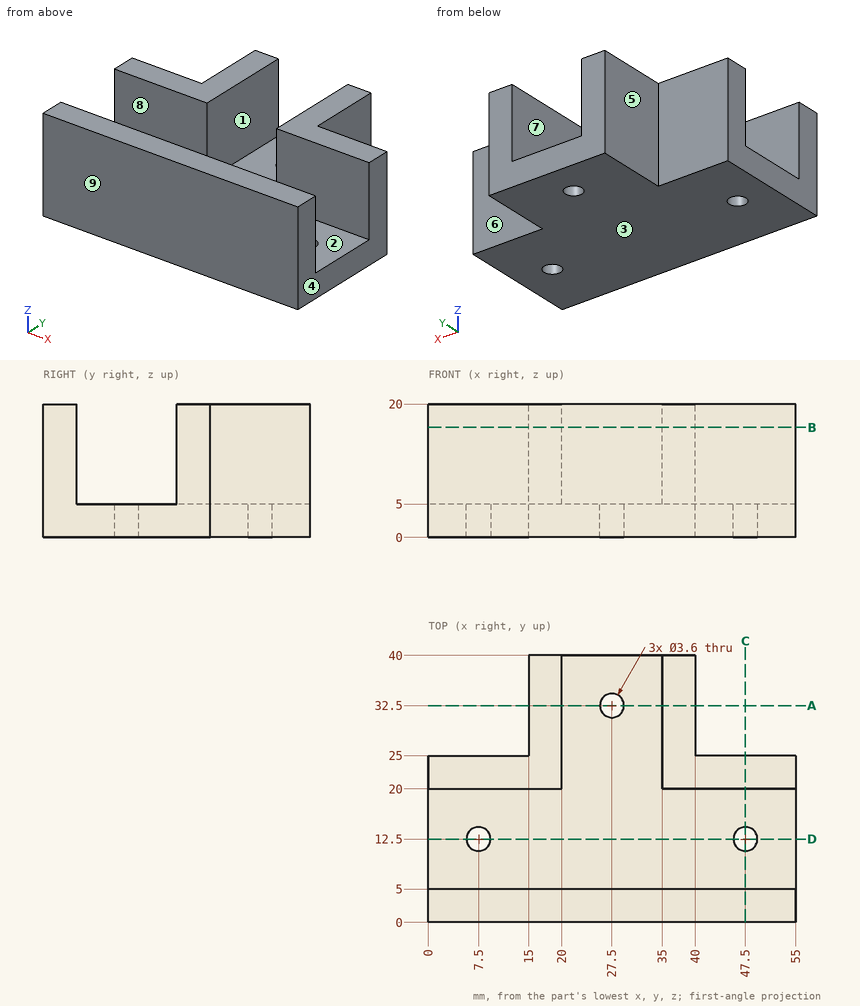
Print and shaded views of the part. All mm, measured from the part's lowest x, y and z. A direction names the side the tool comes from. Coordinates: 2 decimals unless noted, no trailing zeros. Order: outer loops, then holes, each group sorted by start corner. A loop starts at its lowest first (then second) coordinate and runs counter-clockwise, first axis right, second up.
(1) Pull direction X, two halves, no side cores. Call the marked faces 1, 2, 3 and 4: pulls with the +X half, pulls with the -X half, needs draft (parallel to the pull), parting line crosses it, or undercut.
Check sheet entries:
face 1: undercut
face 2: undercut
face 3: needs draft
face 4: pulls with the +X half
(2) Pin check, flat tips, straight feed: pin 1 Ø7.5 at (y, z) = (36, 10) entering from -X; pin 2 Ø4.5 at (x, z) = (11, 5) entering from +Y; pin 3 Ø2 at (x, z) = (32.5, 8) entering from +Y; pin 4 Ø2 at (x, y) = (7.5, 12.5) entering from +Z. Stop position of each tip, or through.
Check sheet entries:
pin 1: stops at x = 15
pin 2: stops at y = 25
pin 3: stops at y = 5
pin 4: passes through
(3) Tool access for the marked faces 5, 6, 7, 8 and 9: list every direction of +Z, -Z, +X, -X, +Y, -Y with a clear straight run to the whole face (end or side of a thin tool).
Check sheet entries:
face 5: +Z, -Z, -X, +Y
face 6: +Z, -Z, +X, +Y
face 7: +Z, +Y
face 8: +Z, +X, -X
face 9: +Z, -Z, +X, -X, -Y
(4) Slice it at A-A, the plane y = 32.5. Write the cut outline in (x, z).
Check sheet entries:
outline: (15, 0) - (25.7, 0) - (25.7, 5) - (20, 5) - (20, 20) - (15, 20) - close; (29.3, 0) - (40, 0) - (40, 20) - (35, 20) - (35, 5) - (29.3, 5) - close
(5) Probe L1, parallel to Y at x = 7.5, z = 3.25; L2, parallel to Y at x = 37.5, z = 13.5; L3, parallel to X at y = 23, z = 11.5. List the from-to ranges inside material, lowest first.
Check sheet entries:
L1: y = 0 to 10.7, 14.3 to 25
L2: y = 0 to 5, 20 to 40
L3: x = 0 to 20, 35 to 55
(6) Slice it at D-D, the plane y = 12.5. Write the cut outline in (x, z).
Check sheet entries:
outline: (0, 0) - (5.7, 0) - (5.7, 5) - (0, 5) - close; (9.3, 0) - (45.7, 0) - (45.7, 5) - (9.3, 5) - close; (49.3, 0) - (55, 0) - (55, 5) - (49.3, 5) - close
(7) Slice it at C-C, the plane x = 47.5. Write the cut outline in (y, z).
Check sheet entries:
outline: (0, 0) - (10.7, 0) - (10.7, 5) - (5, 5) - (5, 20) - (0, 20) - close; (14.3, 0) - (25, 0) - (25, 20) - (20, 20) - (20, 5) - (14.3, 5) - close
(8) Slice it at B-B, the plane z = 16.5. Write the cut outline in (x, y), and give its area (3 significant figures).
Check sheet entries:
outline: (0, 0) - (55, 0) - (55, 5) - (0, 5) - close; (0, 20) - (20, 20) - (20, 40) - (15, 40) - (15, 25) - (0, 25) - close; (35, 20) - (55, 20) - (55, 25) - (40, 25) - (40, 40) - (35, 40) - close
area: 625 mm2
